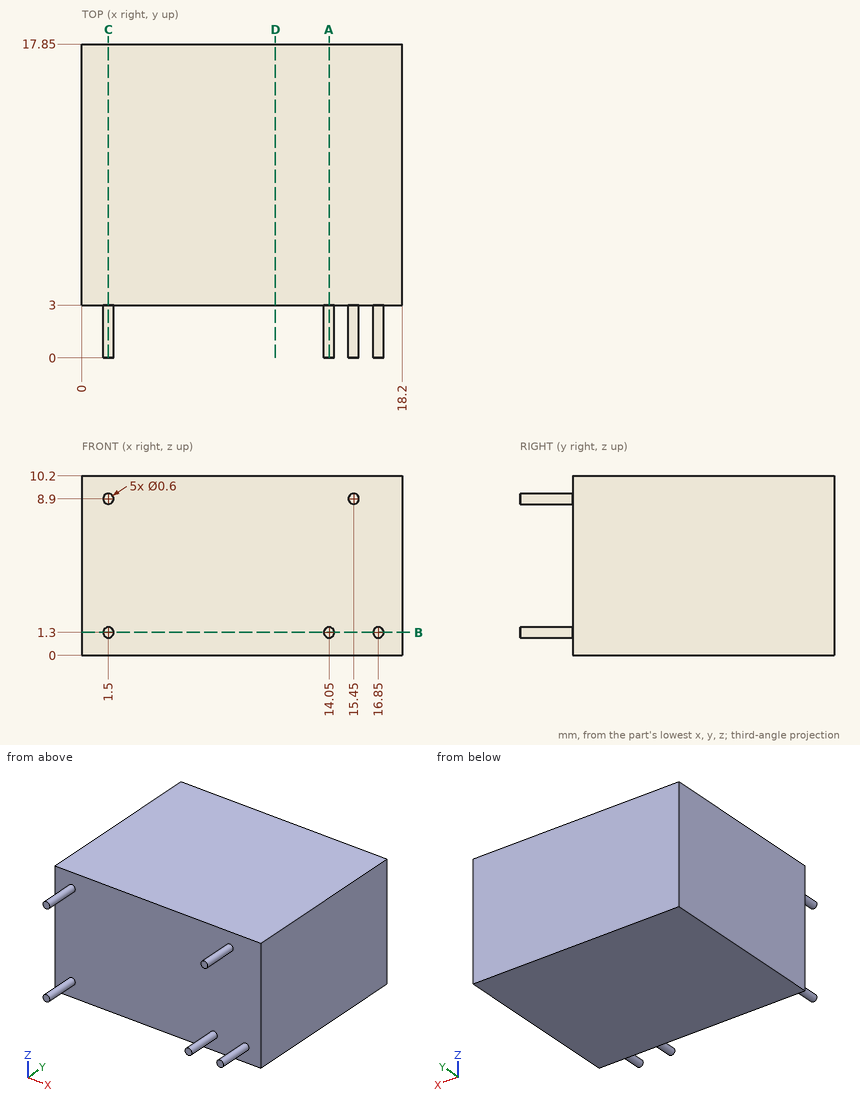
Job drawing, mm, ordinate dimensions from the low corner. One solid piece. Coordinates: 2 decimals unless noted, no trailing zeros. Write each loop counter-clockwise with the first axis right and the second up, starting at its lowest first coordinate (ties: lowest second). Pieces come first, ordered by that corner, then holes. Notation, with made-up numbers: (55.5, 14) -> (72.5, 14) arc R21 ccw to (72.5, 24) -> close; hole circle Ø4 at (-31.5, -10.5). An arc over 180 degrees is marked (long way). Use CSV: the item, a comma, the result in double quotes. Start each with the question number.
Item 1: Band-saw the part on D-D, the plane x = 11. Write the cut outline in (y, z), plus the area to 3 significant figures.
Item 2: Band-saw the part on C-C, the plane x = 1.5. Write the cut outline in (y, z).
Item 3: Band-saw the part on A-A, the plane x = 14.05. Write the cut outline in (y, z).
Item 4: Wall check: probe 1 along Y at (x, z) = (12.75, 7.5). Give the ranges that are in metal, low to high.
Item 5: Band-saw the part on B-B, the plane z = 1.3. Write the cut outline in (x, y).
Item 6: Drop a flat-ended pin along its axis: P1, Ø3, axis at x = 7.5, z = 7.5, coming from the -Y side. Give the stop position or say it passes through.
Response values:
1,outline,"(3, 0) -> (17.85, 0) -> (17.85, 10.2) -> (3, 10.2) -> close"
1,area,"151 mm2"
2,outline,"(0, 1) -> (3, 1) -> (3, 0) -> (17.85, 0) -> (17.85, 10.2) -> (3, 10.2) -> (3, 9.2) -> (0, 9.2) -> (0, 8.6) -> (3, 8.6) -> (3, 1.6) -> (0, 1.6) -> close"
3,outline,"(0, 1) -> (3, 1) -> (3, 0) -> (17.85, 0) -> (17.85, 10.2) -> (3, 10.2) -> (3, 1.6) -> (0, 1.6) -> close"
4,probe 1,"y = 3 to 17.85"
5,outline,"(0, 3) -> (1.2, 3) -> (1.2, 0) -> (1.8, 0) -> (1.8, 3) -> (13.75, 3) -> (13.75, 0) -> (14.35, 0) -> (14.35, 3) -> (16.55, 3) -> (16.55, 0) -> (17.15, 0) -> (17.15, 3) -> (18.2, 3) -> (18.2, 17.85) -> (0, 17.85) -> close"
6,P1,"stops at y = 3"
